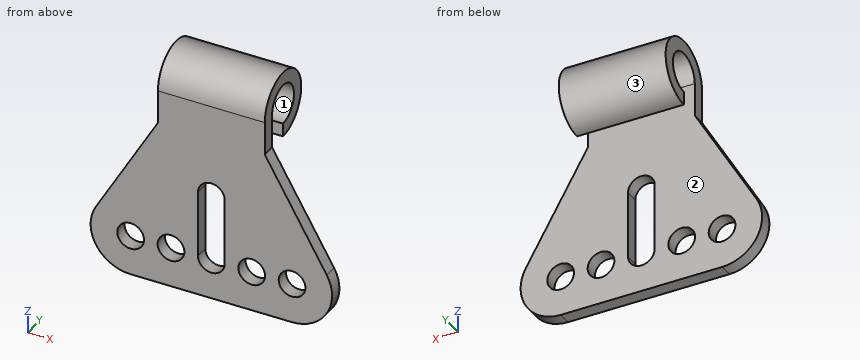
```python
from build123d import *

# Parameters (mm, degrees)
SKETCH_1_R             = 2
SM_BASE_FLANGE_1_DEPTH = 2
OTHER_START            = -8
OTHER_1_DEPTH          = 16


# Read off the part's stored shape, not the designer's step: 褶边1
# Sheet-metal steps are written as plain solids
with BuildPart() as part:
    # Sketch 1 → 基体-法兰1 (new body)
    with BuildSketch(Plane(origin=(0, 0, 0), x_dir=(1, 0, 0), z_dir=(0, 1, 0))):
        with BuildLine():
            Line((-12.083833912, 25), (12.083833912, 25))
            ThreePointArc((12.083833912, 25), (17.282961302, 21.994841295), (17.274021048, 15.989691461))
            Line((17.274021048, 15.989691461), (8, 0))
            Line((8, 0), (8, -5))
            Line((8, -5), (-8, -5))
            Line((-8, -5), (-8, 0))
            Line((-8, 0), (-17.274021048, 15.989691461))
            ThreePointArc((-17.274021048, 15.989691461), (-17.282961302, 21.994841295), (-12.083833912, 25))
        make_face()
        with Locations(Location((-12.083833912, 19, 0), (0, 0, 270))):
            Circle(SKETCH_1_R, mode=Mode.SUBTRACT)
        with Locations(Location((-6.041916956, 19, 0), (0, 0, 270))):
            Circle(SKETCH_1_R, mode=Mode.SUBTRACT)
        with Locations(Location((6.041916956, 19, 0), (0, 0, 270))):
            Circle(SKETCH_1_R, mode=Mode.SUBTRACT)
        with Locations(Location((12.083833912, 19, 0), (0, 0, 270))):
            Circle(SKETCH_1_R, mode=Mode.SUBTRACT)
        with BuildLine():
            Line((-2, 19), (-2, 9))
            ThreePointArc((-2, 9), (0, 7), (2, 9))
            Line((2, 9), (2, 19))
            ThreePointArc((2, 19), (0, 21), (-2, 19))
        make_face(mode=Mode.SUBTRACT)
    extrude(amount=SM_BASE_FLANGE_1_DEPTH)

    # Other 1 outline → Other 1 (add)
    with BuildSketch(Plane.YZ.offset(OTHER_START)):
        with BuildLine():
            Line((5, 2), (5, 0))
            ThreePointArc((5, 0), (8.535533906, 8.535533906), (0, 5))
            Line((0, 5), (2, 5))
            ThreePointArc((2, 5), (7.121320344, 7.121320344), (5, 2))
        make_face()
    extrude(amount=OTHER_1_DEPTH)


solid = part.part
```
The listing builds one solid part. Answer for the finished solid, in the listing's coordinates (mm). Face numbers are marked on the shaded views. Coordinates: 2 decimals unless noted, no trailing zeros. Write each loop counter-clockwise with the first axis right and the second up, starting at its lowest first coordinate (ties: lowest second). Pieces come first, ordered by that corner, then holes.
Q1. The mould has two halves that part along Z. Classify the marked faces 1, 2 and 3: released by +Z, released by -Z, zero draft, split by the parting line, or undercut.
Returned:
face 1: undercut
face 2: zero draft
face 3: split by the parting line
Q2. Section A-A, the plane x = 0 is taken. Write down the section's boundary in (y, z).
Returned:
outline: (0, -25) - (2, -25) - (2, -21) - (0, -21) - close; (0, -7) - (2, -7) - (2, 5) arc R3 cw (long way) to (5, 2) - (5, 0) arc R5 ccw (long way) to (0, 5) - close
Q3. Section D-D, the plane z = -17.5 is taken. Write down the section's boundary in (x, y).
Returned:
outline: (-17.89, 0) - (-13.41, 0) - (-13.41, 2) - (-17.89, 2) - close; (-10.76, 0) - (-7.36, 0) - (-7.36, 2) - (-10.76, 2) - close; (-4.72, 0) - (-2, 0) - (-2, 2) - (-4.72, 2) - close; (2, 0) - (4.72, 0) - (4.72, 2) - (2, 2) - close; (7.36, 0) - (10.76, 0) - (10.76, 2) - (7.36, 2) - close; (13.41, 0) - (17.89, 0) - (17.89, 2) - (13.41, 2) - close
Q4. Section C-C, the plane y = 1 is taken. Write down the section's boundary in (x, z).
Returned:
outline: (-17.27, -15.99) arc R6 ccw to (-12.08, -25) - (12.08, -25) arc R6 ccw to (17.27, -15.99) - (8, 0) - (8, 8) - (-8, 8) - (-8, 0) - close; hole circle Ø4 at (-12.08, -19); hole circle Ø4 at (-6.04, -19); hole (-2, -19) arc R2 ccw to (2, -19) - (2, -9) arc R2 ccw to (-2, -9) - close; hole circle Ø4 at (6.04, -19); hole circle Ø4 at (12.08, -19)
Q5. Find the intervals of material crossed by line 1 along X through (y, z) = (1.65, -19); line 2 along Y through (x, z) = (1.5, 5); line 3 along X through (y, z) = (0.75, -16), in increasing order.
Returned:
line 1: x = -18.08 to -14.08, -10.08 to -8.04, -4.04 to -2, 2 to 4.04, 8.04 to 10.08, 14.08 to 18.08
line 2: y = 0 to 2, 8 to 10
line 3: x = -17.28 to -2, 2 to 17.28
Q6. Given P1, Ø2, axis at x = -0.5, y = 6, coming from the +Z side; P2, Ø1.5, axis at x = -7.5, z = -21, coming from the +Y side; P3, Ø0.6, axis at y = 1.5, z = -16, coming from the -X side; P4, Ø1.5, axis at y = 1.5, z = -6.5, coming from the +X side (3 decimals), each flat-ended and moving along its own axis, determine where each tip first touches the part or whether it passes through.
Returned:
P1: stops at z = 10
P2: stops at y = 2
P3: stops at x = -17.44
P4: stops at x = 12.205
Q7. Section B-B, the plane z = -13 is taken. Write down the section's boundary in (x, y).
Returned:
outline: (-15.54, 0) - (-2, 0) - (-2, 2) - (-15.54, 2) - close; (2, 0) - (15.54, 0) - (15.54, 2) - (2, 2) - close
